Autodesk Inventor part; units mm, degrees
ref_plane "YZ Plane" through (0, 0, 0) normal (1, 0, 0) x (0, 1, 0)
ref_plane "XZ Plane" through (0, 0, 0) normal (0, 1, 0) x (-1, 0, 0)
ref_plane "XY Plane" through (0, 0, 0) normal (0, 0, 1) x (1, 0, 0)
sketch "Sketch1" plane through (0, 0, 0) normal (1, 0, 0) x (0, 1, 0)
  line L0 (75, 0) -> (75, -38)
  line L1 (75, -38) -> (-20, -38)
  line L2 (-20, -38) -> (-20, 0)
  line L3 (-20, 0) -> (75, 0) construction
  line L4 (75, 0) -> (75, 38)
  line L5 (75, 38) -> (-20, 38)
  line L6 (-20, 38) -> (-20, 0)
  point P0 (0, 0)
  dimension "d0" = 38
  dimension "d3" = 75
  dimension "d4" = 20
extrude "Extrusion1" add sketch "Sketch1" along normal mid plane 50
sketch "Sketch2" plane through (25, 0, 0) normal (1, 0, 0) x (0, 0, -1)
  line L0 (38, 75) -> (-38, 75)
  line L1 (-38, 75) -> (-38, -20)
  line L2 (-38, -20) -> (38, -20)
  line L3 (-32, -20) -> (32, -20)
  line L4 (32, -20) -> (32, 63)
  line L5 (32, 63) -> (-32, 63)
  line L6 (-32, 63) -> (-32, -20)
  line L7 (0, 63) -> (0, -20) construction
  point P0 (0, 0)
  dimension "d7" = 6
  dimension "d8" = 12
extrude "Extrusion2" cut sketch "Sketch2" against normal through all
sketch "Sketch3" plane through (-25, -20, 38) normal (0, 0, 1) x (1, 0, 0)
  circle A0 centre (25, 20) radius 10
  dimension "d11" = 20
extrude "Extrusion3" cut sketch "Sketch3" against normal through all
sketch "Sketch4" plane through (-25, 75, 38) normal (0, 1, 0) x (1, 0, 0)
  circle A0 centre (25, 38) radius 10
  dimension "d15" = 20
extrude "Extrusion4" cut sketch "Sketch4" against normal through all
move or copy body "Move Body1" bodies to move or copy 1 copy no rotation origin (0, 0, 0) rotation axis (1, 0, 0) rotation angle 90
move or copy body "Move Body2" bodies to move or copy 1 copy no rotation origin (0, 0, 0) rotation axis (0, 0, 1) rotation angle 90
properties part number "HipYaw_v2"
The listing builds one solid part. Answer for the finished solid, in the listing's coordinates (mm). A direction names the side the tool comes from. Round coordinates to 2 decimals unless told otherwise and drop trailing zeros. Write each loop counter-clockwise with the first axis right and the second up, starting at its lowest first coordinate (ties: lowest second). Pieces come first, ordered by that corner, then holes. Notation, with made-up numbers: (80, -33) -> (120, -33) arc R23 ccw to (120, -17) -> close; hole circle Ø3 at (38, -32). An arc over 180 degrees is marked (long way). Use CSV: the item, a comma, the result in double quotes. Start each with the question number.
(1) Which of the six approach directions +Z, -Z, +X, -X, +Y, -Y give full straight-line access (tool end or side, diameter ignored) to faces 5 (the face through (35, 0, -20)), 6 (the face through (-32, 0, 21))?
(2) Section B-B on z = 0 is taken. Give the vertices of the cut face in (x, y).
(3) Section A-A on x = 0 is taken. Give the vertices of the cut face in (y, z).
(4) Section C-C on z = 43.5 is taken. Give the vertices of the cut face in (x, y).
(5) Section D-D on y = 0 is taken. Give the vertices of the cut face in (x, z).
(6) Consider L1, parallel to X at y = 22.5, z = 47; L2, parallel to Y at x = 0, z = 68; L3, parallel to Z at x = -36.6, y = 0. Determine where each line is inside the solid, lowest interval first. Write a range as from..to.
(7) The mould has two halves that part along X. Classify faces 1 (the face through (9.76, -2.17, 69.08)), 2 (the face through (38, 0, 28)), 3 (the face through (9, -6, 75)), 4 (the face through (-38, 0, 28)): released by +X, released by -X, zero draft, split by the parting line, or undercut.
A:
1,face 5,"-Z, +X, -X, +Y, -Y"
1,face 6,"-Z, +Y, -Y"
2,outline,"(-38, -25) -> (-32, -25) -> (-32, -10) -> (-38, -10) -> close; (-38, 10) -> (-32, 10) -> (-32, 25) -> (-38, 25) -> close; (32, -25) -> (38, -25) -> (38, -10) -> (32, -10) -> close; (32, 10) -> (38, 10) -> (38, 25) -> (32, 25) -> close"
3,outline,"(-25, 63) -> (-10, 63) -> (-10, 75) -> (-25, 75) -> close; (10, 63) -> (25, 63) -> (25, 75) -> (10, 75) -> close"
4,outline,"(-38, -25) -> (-32, -25) -> (-32, 25) -> (-38, 25) -> close; (32, -25) -> (38, -25) -> (38, 25) -> (32, 25) -> close"
5,outline,"(-38, -20) -> (-32, -20) -> (-32, -10) -> (-38, -10) -> close; (-38, 10) -> (-32, 10) -> (-32, 63) -> (-10, 63) -> (-10, 75) -> (-38, 75) -> close; (10, 63) -> (32, 63) -> (32, 10) -> (38, 10) -> (38, 75) -> (10, 75) -> close; (32, -20) -> (38, -20) -> (38, -10) -> (32, -10) -> close"
6,L1,"x = -38..-32, 32..38"
6,L2,"y = -25..-10, 10..25"
6,L3,"z = -20..-10, 10..75"
7,face 1,"undercut"
7,face 2,"released by +X"
7,face 3,"zero draft"
7,face 4,"released by -X"
